Build history of the part. All positions in model axes, mm. A direction names the side the tool comes from. Give positions to 0.01 mm unless a question says otherwise; leave off trailing zeros. Order: outer loops, then holes, each group sorted by start corner. A loop starts at its lowest first (then second) coordinate and runs counter-clockwise, first axis right, second up. Notation, with made-up numbers: (86.25, 14) - (127.25, 14) arc R28 cw to (127.25, 41) - close; hole circle Ø6 at (-3.75, 49). An arc over 180 degrees is marked (long way). Write each question's results on one line, items separated by ' | '. Start each with the question number.
from build123d import *

# Parameters (mm, degrees)
BOSS_EXTRUDE1_DEPTH = 127
SKETCH2_R           = 6.35
CHAMFER1_SIZE       = 0.8


with BuildPart() as part:
    # Sketch1 → Boss-Extrude1 (new body)
    with BuildSketch(Plane(origin=(0, 0, 0), x_dir=(1, 0, 0), z_dir=(0, 1, 0))):
        Polygon((-12.7, 2.667), (12.7, 2.667), (12.7, -2.667), (-12.7, -2.667), (-12.7, -5.867), (15.9, -5.867), (15.9, 5.867), (-12.7, 5.867), align=None)
    extrude(amount=BOSS_EXTRUDE1_DEPTH)

    # Sweep1: sweep along a curve in space
    with BuildLine() as sweep1_path:
        Line((6.375, 9.525, 5.867), (6.375, 9.525, 24.917))
        ThreePointArc((6.375, 9.525, 24.917), (6.375, 13.244743879, 33.897256121), (6.375, 22.225, 37.617))
        Line((6.375, 22.225, 37.617), (6.375, 104.775, 37.617))
        ThreePointArc((6.375, 104.775, 37.617), (6.375, 113.755256121, 33.897256121), (6.375, 117.475, 24.917))
        Line((6.375, 117.475, 24.917), (6.375, 117.475, 5.867))
    # Sketch2 → Sweep1 (sweep)
    with BuildSketch(Plane.XY.offset(5.867)):
        with Locations((6.375, 9.525)):
            Circle(SKETCH2_R)
    sweep(path=sweep1_path.line)

    # Chamfer1
    chamfer1_edges = [part.edges().sort_by_distance(p)[0] for p in [
        (-12.7, 63.5, -5.867),
        (15.9, 63.5, -5.867),
        (15.9, 63.5, 5.867),
        (-12.7, 63.5, 5.867),
        (-12.7, 63.5, 2.667),
        (-12.7, 63.5, -2.667),
        (1.6, 127, 5.867),
        (0.025, 9.525, 5.867),
        (0.025, 117.475, 5.867),
        (15.9, 127, 0),
        (1.6, 127, -5.867),
        (1.6, 0, -5.867),
        (15.9, 0, 0),
        (1.6, 0, 5.867),
    ]]
    chamfer(chamfer1_edges, length=CHAMFER1_SIZE)


with BuildPart() as body_2:
    # Mirror3: mirrored copy
    add(part.part.mirror(Plane(origin=(0, 0, 0), x_dir=(0, 0, 1), z_dir=(1, 0, 0))))


solid = body_2.part
Item 1: Cut at D-D, the plane z = 9. List the corners of the cut face in (x, y) (3 decimals).
Item 2: Cut at C-C, the plane x = -5. Count the separate pieces of the cut face and the enclosed holes in it, then the cut area to 3 significant figures.
Item 3: Two-plate mould, pull along Y, no slides. Class faces 4 (the flat face through (-1, 127, -3)), 5 (the flat face through (-1, 63, 2.667)), 6 (the flat face through (-1, 0, -3)), 7 (the cylindrical face through (-5.55, 111.18, 15.66)): +Y half, -Y half, draft (parallel to the pull), parting line (faces both ways), or undercut.
Item 4: Probe line 1 along Z through (x, y) = (0.5, 102); line 2 along Z through (x, y) = (-4.5, 36); line 3 along Z through (x, y) = (-9, 65.5). List the from-to ranges inside material, lowest first. Write a range as from..to.
Item 5: Flat gauge pins, fed straight in: pin 1 Ø8 at (x, y) = (0.5, 33.5) entering from +Z; pin 2 Ø1 at (x, y) = (4, 96.5) entering from +Z; pin 3 Ø2.5 at (y, z) = (33, -1) entering from +X; pin 4 Ø1.5 at (x, z) = (-8.5, 0) entering from +Y. Where does each tip first touch, or does it go through?
Item 6: Cut at B-B, the plane y = 77.5. List the corners of the cut face in (x, z) (3 decimals).
Item 7: Which spindle directions (+Z, -Z, +X, -X, +Y, -Y) get a long thin tool onto all of the face, cutting with end or side? Do faces 1 (the flat face through (-15.9, 63, 0)), 2 (the cylindrical face through (-4.998, 64.078, 43.816)), 3 (the flat face through (0, 63, -2.667)). Say none if no direction does.
Item 8: Cut at A-A, the plane x = 7.5. List the corners of the cut face in (y, z), then the cut area to 3 significant figures.
Values found:
1) outline: circle Ø12.7 at (-6.375, 9.525); circle Ø12.7 at (-6.375, 117.475)
2) separate pieces: 2 | enclosed holes: 1 | area: 2,800 mm2
3) face 4: +Y half | face 5: draft | face 6: -Y half | face 7: undercut
4) line 1: z = -5.87..-2.67, 2.67..5.87 | line 2: z = -5.87..-2.67, 2.67..5.87, 31.55..43.68 | line 3: z = -5.87..-2.67, 2.67..5.87, 31.83..43.4
5) pin 1: stops at z = 43.28 | pin 2: stops at z = 5.87 | pin 3: stops at x = -12.7 | pin 4: passes through
6) outline: (-15.9, -5.067) - (-15.1, -5.867) - (11.9, -5.867) - (12.7, -5.067) - (12.7, -3.467) - (11.9, -2.667) - (-12.7, -2.667) - (-12.7, 2.667) - (11.9, 2.667) - (12.7, 3.467) - (12.7, 5.067) - (11.9, 5.867) - (-15.1, 5.867) - (-15.9, 5.067) - close; circle Ø12.7 at (-6.375, 37.617)
7) face 1: +Z, -Z, -X, +Y, -Y | face 2: none | face 3: +X, +Y, -Y
8) outline: (0, -5.07) - (0.8, -5.87) - (126.2, -5.87) - (127, -5.07) - (127, -2.67) - (0, -2.67) - close; (0, 2.67) - (127, 2.67) - (127, 5.07) - (126.2, 5.87) - (0.8, 5.87) - (0, 5.07) - close | area: 812 mm2
